Check sheet for the modelled part. Datum: model origin and axes. Units: mm. Face numbers are marked on the shaded views. A direction names the side the tool comes from. Give positions to 0.01 mm unless a question says otherwise; leave off trailing zeros. Loops run counter-clockwise (first coordinate to the right, second up) from the corner with the lowest first, then second, coordinate; pieces in that order, holes last. Notation, with made-up numbers: (80.25, 3.5) - (111.25, 3.5) arc R17 cw to (111.25, 24.5) - close; hole circle Ø7 at (25.25, 61). An arc over 180 degrees is marked (long way). Use one line per item in the form item = value.
from build123d import *

# Parameters (mm, degrees)
RESSALTO_EXTRUS_O1_DEPTH                             = 6
ESBO_O2_W                                            = 18
ESBO_O2_H                                            = 6
RESSALTO_EXTRUS_O2_DEPTH                             = 27
FILETE1_R                                            = 3
ESBO_O4_R                                            = 6
CORTE_EXTRUS_O1_DEPTH                                = 33
ESCAREADO_PARA_PARAFUSO_DE_M_QUINA_COM_C_D           = 2.4
ESCAREADO_PARA_PARAFUSO_DE_M_QUINA_COM_C_CSINK_D     = 4.4
ESCAREADO_PARA_PARAFUSO_DE_M_QUINA_COM_C_CSINK_ANGLE = 90
PADR_OCIRCULAR1_COUNT                                = 3


with BuildPart() as part:
    # Esboço1 → Ressalto-extrusão1 (new body)
    with BuildSketch(Plane.XY):
        with BuildLine():
            Line((-9, 30), (-9, 0))
            Line((-9, 0), (9, 0))
            Line((9, 0), (9, 30))
            Line((9, 30), (5.358457271, 45.739732099))
            ThreePointArc((5.358457271, 45.739732099), (0, 50), (-5.358457271, 45.739732099))
            Line((-5.358457271, 45.739732099), (-9, 30))
        make_face()
    extrude(amount=RESSALTO_EXTRUS_O1_DEPTH)

    # Esboço2 → Ressalto-extrusão2 (add)
    with BuildSketch(Plane.XY.offset(6)):
        with Locations((0, 3)):
            Rectangle(ESBO_O2_W, ESBO_O2_H)
    extrude(amount=RESSALTO_EXTRUS_O2_DEPTH)

    # Filete1
    filete1_edges = [part.edges().sort_by_distance(p)[0] for p in [
        (0, 6, 6),
        (0, 0, 0),
    ]]
    fillet(filete1_edges, radius=FILETE1_R)

    # Esboço4 → Corte-extrusão1 (cut)
    with BuildSketch(Plane(origin=(0, 0, 0), x_dir=(-1, 0, 0), z_dir=(0, 0, -1))):
        with Locations((0, 13)):
            Circle(ESBO_O4_R)
    extrude(amount=-CORTE_EXTRUS_O1_DEPTH, mode=Mode.SUBTRACT)

    # Escareado para parafuso de máquina com cabeça chata de M22 (through all)
    with Locations(Plane(origin=(0, 47.5, 6), x_dir=(1, 0, 0), z_dir=(0, 0, 1))):
        with Locations((0, 0)):
            escareado_para_parafuso_de_m_quina_com_c = CounterSinkHole(ESCAREADO_PARA_PARAFUSO_DE_M_QUINA_COM_C_D / 2, ESCAREADO_PARA_PARAFUSO_DE_M_QUINA_COM_C_CSINK_D / 2, counter_sink_angle=ESCAREADO_PARA_PARAFUSO_DE_M_QUINA_COM_C_CSINK_ANGLE)

    # PadrãoCircular1: Escareado para parafuso de máquina com cabeça chata de M22 ×3 about axis
    padr_ocircular1_axis = Axis((0, 44.5, 0), (0, 0, 1))
    for i in range(1, PADR_OCIRCULAR1_COUNT):
        add(escareado_para_parafuso_de_m_quina_com_c.rotate(padr_ocircular1_axis, i * 360 / PADR_OCIRCULAR1_COUNT), mode=Mode.SUBTRACT)


solid = part.part
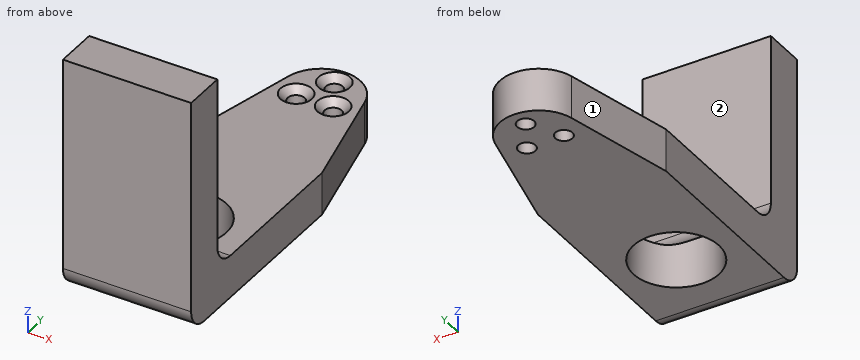
Item 1: Gauge pin test, flat ends, axial feed: P1, Ø2, axis at x = -1, y = 34.5, coming from the +Z side; P2, Ø1.9, axis at x = -2.6, y = 43, coming from the +Z side; P3, Ø5.5, axis at x = -0.5, z = 23, coming from the +Y side. Record the tip position at first contact, or that the pin passes through.
Answer block:
P1 = 6
P2 = through
P3 = 6
Item 2: Section check A-A on y = 13. Record the boundary of the cut face in (x, z).
Answer block:
outline = (-9, 0) - (-6, 0) - (-6, 6) - (-9, 6) - close; (6, 0) - (9, 0) - (9, 6) - (6, 6) - close
Item 3: Thickness scan on L1, parallel to X at y = 43, z = 2.3; L2, parallel to Y at x = -0.5, z = 3; L3, parallel to Y at x = 3, z = 16. Record the ranges inside material, lowest first.
Answer block:
L1 = -5.99 to -3.8, -1.4 to 1.4, 3.8 to 5.99
L2 = 0 to 7.02, 18.98 to 46.41, 48.59 to 49.98
L3 = 0 to 6
Item 4: Section check B-B on y = 43. Record the boundary of the cut face in (x, z).
Answer block:
outline = (-5.99, 0) - (-3.8, 0) - (-3.8, 5) - (-4.8, 6) - (-5.99, 6) - close; (-1.4, 0) - (1.4, 0) - (1.4, 5) - (0.4, 6) - (-0.4, 6) - (-1.4, 5) - close; (3.8, 0) - (5.99, 0) - (5.99, 6) - (4.8, 6) - (3.8, 5) - close
Item 5: Section check D-D on y = 26. Record the boundary of the cut face in (x, z), then the cut area to 3 significant figures.
Answer block:
outline = (-9, 0) - (9, 0) - (9, 6) - (-9, 6) - close
area = 108 mm2
Item 6: Section check C-C on x = 6.75. Record the boundary of the cut face in (y, z), then the cut area to 3 significant figures.
Answer block:
outline = (0, 3) arc R3 ccw to (3, 0) - (39.73, 0) - (39.73, 6) - (9, 6) arc R3 cw to (6, 9) - (6, 33) - (0, 33) - close
area = 400 mm2
Item 7: Access from +Z, -Z, +X, -X, +Y, -Y to the whole of each face (thin tool, end or side, straight path). Record for the marked faces 1 and 2.
Answer block:
face_1 = +Z, -Z, -X, +Y
face_2 = +Z, +X, -X, +Y
